CAD build for the part. Positions are in the model's coordinates, mm. A direction names the side the tool comes from. Give positions to 0.01 mm unless a question says otherwise; leave off trailing zeros. Write each loop counter-clockwise with the first axis right and the second up, starting at its lowest first coordinate (ties: lowest second). Pieces come first, ordered by that corner, then holes. Notation, with made-up numbers: (76, 19.25) - (131, 19.25) arc R18 cw to (131, 43.25) - close; hole circle Ø6 at (57, 62). An arc over 180 degrees is marked (long way). Write item = value, one per line. Start each with the question number.
```python
from build123d import *

# Parameters (mm, degrees)
F0_W    = 10
F0_H    = 5
F0_H_2  = 3
F2_SIZE = 2


with BuildPart() as f1:
    # F0 (on Front) → F1 (revolve)
    with BuildSketch(Plane.XZ):
        with Locations((-5, 2.5)):
            Rectangle(F0_W, F0_H)
        Polygon((-10, 0), (-10, 5), (-13.464102, 3), (-13.464102, 0), align=None)
        with Locations((-18.464102, 1.5)):
            Rectangle(F0_W, F0_H_2)
        Polygon((-23.464102, 0), (-23.464102, 3), (-23.464102, 6), (-29.464102, 6), (-29.464102, 0), align=None)
    revolve(axis=Axis((-14.839673, 0, 0), (-1, 0, 0)))

    # F2
    f2_edges = [f1.edges().sort_by_distance(p)[0] for p in [
        (0, 0, -5),
    ]]
    chamfer(f2_edges, length=F2_SIZE)


solid = f1.part
```
1. Mould opens along X. For faces 1 (the cylindrical face through (-18, 0, -3)), 2 (the cylindrical face through (-5.94, -4.88, -1.08)), 3 (the flat face through (-29.464, 0, 0)), 4 (the conical face through (-0.125, -3.051, -0.677)) say: +X half, -X half, draft (parallel to the pull), parting line (faces both ways), or undercut.
2. Pin check, flat tips, straight feed: pin 1 Ø6 at (x, y) = (-18, 0.5) entering from -Z; pin 2 Ø6 at (x, z) = (-11.5, -4.5) entering from -Y; pin 3 Ø5 at (x, z) = (-12, 0.5) entering from -Y. Stop position of each tip, or through.
3. Wall check: line 1 along X through (y, z) = (-3.5, 0); line 2 along X through (y, z) = (3.75, -4.25); line 3 along X through (y, z) = (-1.75, 4.5). Give the ranges that are in metal, low to high.
4. Cut at A-A (y = 0). Give the cut face in (x, z).
5. Cut at D-D (x = -26.5). Give the cut face in (y, z), then the cut area to 3 significant figures.
6. Cut at C-C (x = -2.5). Give the cut face in (y, z), then the cut area to 3 significant figures.
7. Tool access for faces 5 (the cylindrical face through (-27, 0, -6)), 6 (the conical face through (-13.3, -3.02, -0.67)): list every direction of +Z, -Z, +X, -X, +Y, -Y with a clear straight run to the whole face (end or side of a thin tool).
Output:
q1.face_1 = undercut
q1.face_2 = draft
q1.face_3 = -X half
q1.face_4 = +X half
q2.pin_1 = -3
q2.pin_2 = -4.62
q2.pin_3 = -5
q3.line_1 = -29.46 to -23.46, -12.6 to -0.5
q3.line_2 = -29.46 to -23.46
q3.line_3 = -29.46 to -23.46, -10.3 to -1.83
q4.outline = (-29.46, -6) - (-23.46, -6) - (-23.46, -3) - (-13.46, -3) - (-10, -5) - (-2, -5) - (0, -3) - (0, 3) - (-2, 5) - (-10, 5) - (-13.46, 3) - (-23.46, 3) - (-23.46, 6) - (-29.46, 6) - close
q5.outline = circle Ø12 at (0, 0)
q5.area = 113 mm2
q6.outline = circle Ø10 at (0, 0)
q6.area = 78.5 mm2
q7.face_5 = +X, -X
q7.face_6 = none
